Read the model definition and answer for the solid it produces. Units are mm, in the model's axes. Face numbers are marked on the shaded views. Give positions to 0.01 mm unless a question says otherwise; leave off trailing zeros. Write each loop counter-clockwise with the first axis right and the second up, starting at its lowest first coordinate (ties: lowest second). Pieces come first, ordered by that corner, then holes. Notation, with made-up numbers: M 18.5,-0.5 L 61.5,-0.5 A8 cw 61.5,5.5 Z; hole C 67,11 d1. An arc over 180 degrees is marked long. Put each result on its own line as item: value.
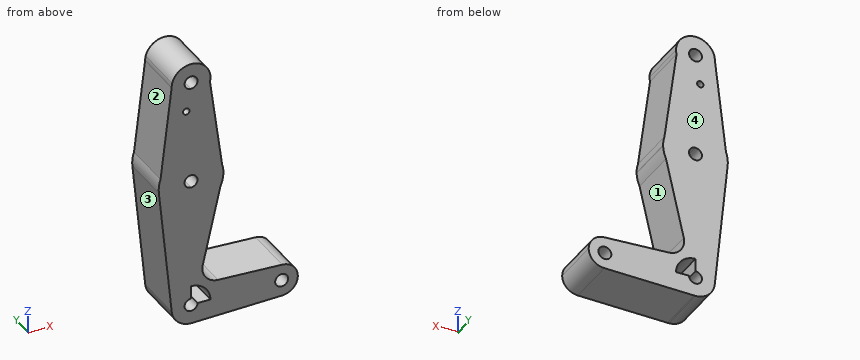
from build123d import *

# Parameters (mm, degrees)
F0_R     = 1.5875
F1_DEPTH = 25.4


with BuildPart() as f1:
    # F0 (on Front) → F1 (new body)
    with BuildSketch(Plane.XZ):
        with BuildLine():
            ThreePointArc((0, 9.525), (-7.063929059, 6.3895642457), (-9.4772553384, -0.9525))
            ThreePointArc((-9.4772553384, -0.9525), (-6.3895642457, -7.063929059), (0, -9.525))
            Line((0, -9.525), (0.6773435479, -9.500885786))
            ThreePointArc((0.6773435479, -9.500885786), (6.9705567315, -6.4912990883), (9.525, 0))
            Line((9.525, 0), (3.175, 0))
            ThreePointArc((3.175, 0), (-2.2450640303, -2.2450640303), (0, 3.175))
            Line((0, 3.175), (0, 9.525))
        make_face()
        with BuildLine():
            Line((-15.7954255641, 61.9125), (-9.4772553384, -0.9525))
            ThreePointArc((-9.4772553384, -0.9525), (-7.063929059, 6.3895642457), (0, 9.525))
            Line((0, 9.525), (0, 47.625))
            ThreePointArc((0, 47.625), (-10.6492737428, 51.7267849017), (-15.7954255641, 61.9125))
        make_face()
        with BuildLine():
            Line((0.6773435479, -9.500885786), (0, -9.525))
            ThreePointArc((0, -9.525), (0.3388863295, -9.5189695375), (0.6773435479, -9.500885786))
        make_face()
        with BuildLine():
            Line((0, 47.625), (0, 9.525))
            ThreePointArc((0, 9.525), (6.7351920908, 6.7351920908), (9.525, 0))
            Line((9.525, 0), (36.5125, 0))
            ThreePointArc((36.5125, 0), (38.9380895153, 5.7116327839), (44.7324052746, 7.9324746146))
            Line((44.7324052746, 7.9324746146), (13.2108551379, 9.0546782715))
            ThreePointArc((13.2108551379, 9.0546782715), (7.1911937291, 12.1538217133), (5.742542983, 18.767627317))
            Line((5.742542983, 18.767627317), (14.4405270392, 56.9055474959))
            ThreePointArc((14.4405270392, 56.9055474959), (8.5827935865, 50.145177678), (0, 47.625))
        make_face()
        with BuildLine():
            Line((-14.9746534016, 68.7702353365), (-15.7954255641, 61.9125))
            ThreePointArc((-15.7954255641, 61.9125), (-10.6492737428, 51.7267849017), (0, 47.625))
            Line((0, 47.625), (0, 60.325))
            ThreePointArc((0, 60.325), (-3.175, 63.5), (0, 66.675))
            Line((0, 66.675), (0, 79.375))
            ThreePointArc((0, 79.375), (-9.1747108683, 76.4553195825), (-14.9746534016, 68.7702353365))
        make_face()
        with BuildLine():
            ThreePointArc((-14.9746534016, 68.7702353365), (-15.7625053013, 65.3865448909), (-15.7954255641, 61.9125))
            Line((-15.7954255641, 61.9125), (-14.9746534016, 68.7702353365))
        make_face()
        with BuildLine():
            ThreePointArc((9.525, 0), (6.9705567315, -6.4912990883), (0.6773435479, -9.500885786))
            Line((0.6773435479, -9.500885786), (44.7324052746, -7.9324746146))
            ThreePointArc((44.7324052746, -7.9324746146), (38.9380895153, -5.7116327839), (36.5125, 0))
            Line((36.5125, 0), (9.525, 0))
        make_face()
        with BuildLine():
            Line((0, 60.325), (0, 47.625))
            ThreePointArc((0, 47.625), (8.5827935865, 50.145177678), (14.4405270392, 56.9055474959))
            Line((14.4405270392, 56.9055474959), (15.8717991204, 63.1812247139))
            Line((15.8717991204, 63.1812247139), (15.2237290867, 68.0004108363))
            ThreePointArc((15.2237290867, 68.0004108363), (9.5018841019, 76.2173040977), (0, 79.375))
            Line((0, 79.375), (0, 66.675))
            ThreePointArc((0, 66.675), (2.2450640303, 65.7450640303), (3.175, 63.5))
            ThreePointArc((3.175, 63.5), (2.2450640303, 61.2549359697), (0, 60.325))
        make_face()
        with BuildLine():
            Line((-9.524999423, 114.3033154892), (-14.9746534016, 68.7702353365))
            ThreePointArc((-14.9746534016, 68.7702353365), (-9.1747108683, 76.4553195825), (0, 79.375))
            Line((0, 79.375), (0, 100.0252))
            Line((0, 100.0252), (0, 104.775))
            ThreePointArc((0, 104.775), (-6.7363641912, 107.5659802137), (-9.524999423, 114.3033154892))
        make_face()
        with Locations((-2.3593854516, 100.0478582527)):
            Circle(F0_R, mode=Mode.SUBTRACT)
        with BuildLine():
            ThreePointArc((36.5125, 0), (38.9380895153, -5.7116327839), (44.7324052746, -7.9324746146))
            ThreePointArc((44.7324052746, -7.9324746146), (50.1616327839, -5.5119104847), (52.3875, 0))
            ThreePointArc((52.3875, 0), (50.1616327839, 5.5119104847), (44.7324052746, 7.9324746146))
            ThreePointArc((44.7324052746, 7.9324746146), (38.9380895153, 5.7116327839), (36.5125, 0))
        make_face()
        with BuildLine():
            ThreePointArc((47.625, 0), (44.45, -3.175), (41.275, 0))
            ThreePointArc((41.275, 0), (44.45, 3.175), (47.625, 0))
        make_face(mode=Mode.SUBTRACT)
        with BuildLine():
            Line((15.8717991204, 63.1812247139), (14.4405270392, 56.9055474959))
            ThreePointArc((14.4405270392, 56.9055474959), (15.4775744365, 59.9700829241), (15.8717991204, 63.1812247139))
        make_face()
        with BuildLine():
            Line((0, 100.0252), (0, 79.375))
            ThreePointArc((0, 79.375), (9.5018841019, 76.2173040977), (15.2237290867, 68.0004108363))
            Line((15.2237290867, 68.0004108363), (9.283878963, 112.1703952479))
            ThreePointArc((9.283878963, 112.1703952479), (5.9346920618, 106.8498285166), (0, 104.775))
            Line((0, 104.775), (0, 100.0252))
        make_face()
        with BuildLine():
            Line((-9.2567511899, 116.5445895858), (-9.524999423, 114.3033154892))
            ThreePointArc((-9.524999423, 114.3033154892), (-6.7363641912, 107.5659802137), (0, 104.775))
            ThreePointArc((0, 104.775), (5.9346920618, 106.8498285166), (9.283878963, 112.1703952479))
            ThreePointArc((9.283878963, 112.1703952479), (9.464527778, 113.2283942242), (9.525, 114.3))
            ThreePointArc((9.525, 114.3), (1.13028092, 123.7577000397), (-9.2567511899, 116.5445895858))
        make_face()
        with BuildLine():
            ThreePointArc((3.175, 114.3), (2.2450640303, 112.0549359697), (0, 111.125))
            ThreePointArc((0, 111.125), (-2.2450640303, 116.5450640303), (3.175, 114.3))
        make_face(mode=Mode.SUBTRACT)
        with BuildLine():
            ThreePointArc((-9.2567511899, 116.5445895858), (-9.4575031808, 115.4319269345), (-9.524999423, 114.3033154892))
            Line((-9.524999423, 114.3033154892), (-9.2567511899, 116.5445895858))
        make_face()
        with BuildLine():
            Line((15.2237290867, 68.0004108363), (15.8717991204, 63.1812247139))
            ThreePointArc((15.8717991204, 63.1812247139), (15.8741997599, 63.340604322), (15.875, 63.5))
            ThreePointArc((15.875, 63.5), (15.7113386484, 65.7736452834), (15.2237290867, 68.0004108363))
        make_face()
    extrude(amount=F1_DEPTH)


solid = f1.part
(1) Straight lines are drawn through the part: line 1 along Z through (x, y) = (44.45, -17.25) (3 decimals); line 2 along X through (y, z) = (-16, 114.3) (3 decimals); line 3 along Z through (x, y) = (2, -11.5). For each, find the intervals that lie inside material, in ascending order. Write a range as from..to.
Result:
line 1: z = -7.943..-3.175, 3.175..7.943
line 2: x = -9.525..-3.175, 3.175..9.525
line 3: z = -9.45..-2.47, 9.31..61.03, 65.97..111.83, 116.77..123.61
(2) For a pull along Z with two mould halves and no side action, classify the marked faces 1, 2, 3 and 4 as +Z half, -Z half, draft (parallel to the pull), parting line (faces both ways), or undercut.
Result:
face 1: undercut
face 2: +Z half
face 3: -Z half
face 4: draft
(3) Section C-C on z = 74 is taken. Determine the outline of the cut face in (x, y).
Result:
outline: M -14.35,-25.4 L 14.42,-25.4 L 14.42,0 L -14.35,0 Z
(4) Section B-B on y = -2 is taken. Give the number of separate pieces and of enclosed holes in the cut face, and give its area (3 significant figures).
Result:
separate pieces: 1
enclosed holes: 5
area: 3,520 mm²
(5) Given pin 1 Ø1.9 at (x, y) = (6.5, -17) entering from +Z; pin 2 Ø5 at (x, y) = (21.5, -9) entering from +Z; pin 3 Ø1.5 at (x, y) = (27, -21) entering from -Z; pin 4 Ø10 at (x, z) = (11.5, 19) entering from +Y, each flat-ended and moving along its own axis, determine where each tip first touches the part or whether it passes through.
Result:
pin 1: stops at z = 122.04
pin 2: stops at z = 8.85
pin 3: stops at z = -8.59
pin 4: passes through
(6) Section D-D on x = 34 is taken. Determine the outline of the cut face in (y, z), and give its area (3 significant figures).
Result:
outline: M -25.4,-8.31 L 0,-8.31 L 0,8.31 L -25.4,8.31 Z
area: 422 mm²
(7) Section A-A on x = 8 is taken. Determine the outline of the cut face in (y, z), and give its area (3 significant figures).
Result:
outline: M -25.4,-9.24 L 0,-9.24 L 0,0 L -25.4,0 Z; M -25.4,5.17 L 0,5.17 L 0,11.25 L -25.4,11.25 Z; M -25.4,28.67 L 0,28.67 L 0,119.47 L -25.4,119.47 Z
area: 2,700 mm²
